Geometry check sheet. Reference: the model listing, model coordinates, mm. Give positions to 0.01 mm unless a question says otherwise; leave off trailing zeros. Write item = value, one per line. Start each with the question number.
1. Thickness scan on line 1 along Z through (x, y) = (-152.05, 3.75); line 2 along X through (y, z) = (1.5, 0); line 3 along X through (y, z) = (4.5, -33.89). Record the ranges inside material, lowest first.
2. Cross-section at A-A, the plane y = 4.5. State how many separate pieces and enclosed holes the cut face has, plus the area to 3 significant figures.
3. Depth check by flat-ended pin: P1, Ø3.5, axis at x = 51.15, z = 17.312, coming from the -Y side; P2, Ø1.5, axis at x = 51.15, z = -39.688, coming from the +Y side; P3, Ø1.1, axis at x = 241.5, y = 5, coming from the +Z side; P4, Ø1, axis at x = 164.5, y = 1.5, coming from the -Z side. Enter the tip coordinate at first touch or a pass-through.
```python
from build123d import *

# Parameters (mm, degrees)
SKETCH1_W           = 520.0000014
SKETCH1_H           = 87.376
BOSS_EXTRUDE1_DEPTH = 6.35
SKETCH3_W           = 27
SKETCH3_H           = 7.62
CUT_EXTRUDE2_DEPTH  = 7.35
SKETCH6_W           = 12.7
SKETCH6_H           = 72.136
CUT_EXTRUDE5_DEPTH  = 7.35
CHAMFER1_SIZE       = 2.54
SKETCH8_R           = 1.4
CUT_EXTRUDE7_DEPTH  = 7.35
SKETCH9_R           = 2.0499959
CUT_EXTRUDE8_DEPTH  = 7.35
SKETCH10_R          = 1.27
CUT_EXTRUDE9_DEPTH  = 7.35
SKETCH11_R          = 2.05
CUT_EXTRUDE10_DEPTH = 7.35
SKETCH12_R          = 1.27
CUT_EXTRUDE11_DEPTH = 7.35
SKETCH13_W          = 6.35
SKETCH13_H          = 13.335
CUT_EXTRUDE12_DEPTH = 7.35
SKETCH14_R          = 1.6
CUT_EXTRUDE13_DEPTH = 7.35


with BuildPart() as part:
    # Sketch1 → Boss-Extrude1 (new body)
    with BuildSketch(Plane(origin=(0, 0, 0), x_dir=(1, 0, 0), z_dir=(0, 1, 0))):
        Rectangle(SKETCH1_W, SKETCH1_H)
    extrude(amount=BOSS_EXTRUDE1_DEPTH)

    # Sketch3 → Cut-Extrude2 (cut, through all)
    with BuildSketch(Plane(origin=(0, 6.35, 0), x_dir=(1, 0, 0), z_dir=(0, 1, 0))):
        with Locations((-246.5000007, 39.878)):
            Rectangle(SKETCH3_W, SKETCH3_H)
        with Locations((-246.5000007, -39.878)):
            Rectangle(SKETCH3_W, SKETCH3_H)
        with Locations((246.5000007, -39.878)):
            Rectangle(SKETCH3_W, SKETCH3_H)
        with Locations((246.5000007, 39.878)):
            Rectangle(SKETCH3_W, SKETCH3_H)
    extrude(amount=-CUT_EXTRUDE2_DEPTH, mode=Mode.SUBTRACT)

    # Sketch6 → Cut-Extrude5 (cut, through all)
    with BuildSketch(Plane(origin=(0, 6.35, 0), x_dir=(1, 0, 0), z_dir=(0, 1, 0))):
        with Locations((253.6500007, 0)):
            Rectangle(SKETCH6_W, SKETCH6_H)
    extrude(amount=-CUT_EXTRUDE5_DEPTH, mode=Mode.SUBTRACT)

    # Chamfer1
    chamfer1_edges = [part.edges().sort_by_distance(p)[0] for p in [
        (0, 0, -43.688),
        (0, 0, 43.688),
        (240.1500007, 0, -36.068),
        (-246.5000007, 0, 36.068),
        (-246.5000007, 0, -36.068),
        (240.1500007, 0, 36.068),
    ]]
    chamfer(chamfer1_edges, length=CHAMFER1_SIZE)

    # Sketch8 → Cut-Extrude7 (cut, through all)
    with BuildSketch(Plane(origin=(0, 6.35, 0), x_dir=(1, 0, 0), z_dir=(0, 1, 0))):
        with Locations((-219.2000007, 10)):
            Circle(SKETCH8_R)
        with Locations((-219.2000007, -10)):
            Circle(SKETCH8_R)
        with Locations((-195.5000007, 0)):
            Circle(SKETCH8_R)
    extrude(amount=-CUT_EXTRUDE7_DEPTH, mode=Mode.SUBTRACT)

    # Sketch9 → Cut-Extrude8 (cut, through all)
    with BuildSketch(Plane(origin=(0, 6.35, 0), x_dir=(1, 0, 0), z_dir=(0, 1, 0))):
        with Locations((-133.0000007, 33.89)):
            Circle(SKETCH9_R)
        with Locations((-152.0500007, 14.84)):
            Circle(SKETCH9_R)
        with Locations((-152.0500007, -14.84)):
            Circle(SKETCH9_R)
        with Locations((-133.0000007, -33.89)):
            Circle(SKETCH9_R)
        with Locations((16.6799993, 33.89)):
            Circle(SKETCH9_R)
        with Locations((35.7299993, 14.84)):
            Circle(SKETCH9_R)
        with Locations((35.7299993, -14.84)):
            Circle(SKETCH9_R)
        with Locations((16.6799993, -33.89)):
            Circle(SKETCH9_R)
    extrude(amount=-CUT_EXTRUDE8_DEPTH, mode=Mode.SUBTRACT)

    # Sketch10 → Cut-Extrude9 (cut, through all)
    with BuildSketch(Plane(origin=(0, 6.35, 0), x_dir=(1, 0, 0), z_dir=(0, 1, 0))):
        with Locations((-200.3100007, -18.415)):
            Circle(SKETCH10_R)
        with Locations((-215.5500007, -18.415)):
            Circle(SKETCH10_R)
        with Locations((-200.3100007, 18.415)):
            Circle(SKETCH10_R)
        with Locations((-215.5500007, 18.415)):
            Circle(SKETCH10_R)
        with Locations((-185.0700007, 18.415)):
            Circle(SKETCH10_R)
        with Locations((-185.0700007, -18.415)):
            Circle(SKETCH10_R)
    extrude(amount=-CUT_EXTRUDE9_DEPTH, mode=Mode.SUBTRACT)

    # Sketch11 → Cut-Extrude10 (cut, through all)
    with BuildSketch(Plane(origin=(0, 6.35, 0), x_dir=(1, 0, 0), z_dir=(0, 1, 0))):
        with Locations((240.9500007, 0)):
            Circle(SKETCH11_R)
    extrude(amount=-CUT_EXTRUDE10_DEPTH, mode=Mode.SUBTRACT)

    # Sketch12 → Cut-Extrude11 (cut, through all)
    with BuildSketch(Plane(origin=(0, 6.35, 0), x_dir=(1, 0, 0), z_dir=(0, 1, 0))):
        with Locations((51.1499993, 39.688)):
            Circle(SKETCH12_R)
        with Locations((131.1499993, 39.688)):
            Circle(SKETCH12_R)
        with Locations((51.1499993, -17.312)):
            Circle(SKETCH12_R)
        with Locations((131.1499993, -17.312)):
            Circle(SKETCH12_R)
    extrude(amount=-CUT_EXTRUDE11_DEPTH, mode=Mode.SUBTRACT)

    # Sketch13 → Cut-Extrude12 (cut, through all)
    with BuildSketch(Plane(origin=(0, 6.35, 0), x_dir=(1, 0, 0), z_dir=(0, 1, 0))):
        with Locations((244.1250007, -14.605)):
            Rectangle(SKETCH13_W, SKETCH13_H)
        with Locations((244.1250007, 14.605)):
            Rectangle(SKETCH13_W, SKETCH13_H)
    extrude(amount=-CUT_EXTRUDE12_DEPTH, mode=Mode.SUBTRACT)

    # Sketch14 → Cut-Extrude13 (cut, through all)
    with BuildSketch(Plane(origin=(0, 6.35, 0), x_dir=(1, 0, 0), z_dir=(0, 1, 0))):
        with Locations((164.0529993, 15)):
            Circle(SKETCH14_R)
        with Locations((194.0529993, 15)):
            Circle(SKETCH14_R)
        with Locations((164.0529993, -15)):
            Circle(SKETCH14_R)
        with Locations((194.0529993, -15)):
            Circle(SKETCH14_R)
    extrude(amount=-CUT_EXTRUDE13_DEPTH, mode=Mode.SUBTRACT)


solid = part.part
```
Answers:
q1.line_1 = -43.69 to -16.89, -12.79 to 12.79, 16.89 to 43.69
q1.line_2 = -260 to -196.9, -194.1 to 238.9, 243 to 247.3
q1.line_3 = -260 to -135.05, -130.95 to 14.63, 18.73 to 247.3
q2.separate_pieces = 1
q2.enclosed_holes = 26
q2.area = 43,300 mm^2
q3.P1 = 0
q3.P2 = through
q3.P3 = 36.07
q3.P4 = -43.15
